Build history of the part. All positions in model axes, mm. A direction names the side the tool comes from. Round coordinates to 2 decimals unless told otherwise and drop trailing zeros. Write each loop counter-clockwise with the first axis right and the second up, starting at its lowest first coordinate (ties: lowest second). Pieces come first, ordered by that corner, then holes. Notation, with made-up numbers: (80.25, 67.25) -> (89.25, 67.25) arc R19 ccw to (89.25, 86.25) -> close; hole circle Ø4 at (2.25, 41.5). An arc over 180 degrees is marked (long way). Answer as CSV lines item,"result".
from build123d import *

# Parameters (mm, degrees)
SKETCH1_W           = 72.5
SKETCH1_H           = 72.5
SKETCH1_R           = 17.5
SKETCH1_R_2         = 2.125
BOSS_EXTRUDE1_DEPTH = 5
BOSS_EXTRUDE2_DEPTH = 50
SKETCH18_R          = 5
CUT_EXTRUDE1_DEPTH  = 2.5
BOSS_EXTRUDE3_DEPTH = 5.5
SKETCH8_W           = 72.5
SKETCH8_H           = 5
BOSS_EXTRUDE4_DEPTH = 54.5
BOSS_EXTRUDE5_DEPTH = 35
BOSS_EXTRUDE7_DEPTH = 1.25
SKETCH12_W          = 85.832523084
SKETCH12_H          = 136.148140064
SKETCH12_R          = 2.25
BOSS_EXTRUDE6_DEPTH = 5
FILLET10_R          = 0.5
SKETCH26_W          = 72.5
SKETCH26_H          = 36.25
CUT_EXTRUDE3_DEPTH  = 166.204098106


with BuildPart() as part:
    # Sketch1 → Boss-Extrude1 (new body)
    with BuildSketch(Plane.XY):
        with Locations((36.25, 36.25)):
            Rectangle(SKETCH1_W, SKETCH1_H)
        with Locations((36.25, 36.25)):
            Circle(SKETCH1_R, mode=Mode.SUBTRACT)
        with Locations((11.25, 61.25)):
            Circle(SKETCH1_R_2, mode=Mode.SUBTRACT)
        with Locations((61.25, 61.25)):
            Circle(SKETCH1_R_2, mode=Mode.SUBTRACT)
        with Locations((61.25, 11.25)):
            Circle(SKETCH1_R_2, mode=Mode.SUBTRACT)
        with Locations((11.25, 11.25)):
            Circle(SKETCH1_R_2, mode=Mode.SUBTRACT)
    extrude(amount=BOSS_EXTRUDE1_DEPTH)

    # Sketch18 → Cut-Extrude1 (cut)
    with BuildSketch(Plane.XY):
        with Locations((61.25, 61.25)):
            Circle(SKETCH18_R)
        with Locations((11.25, 61.25)):
            Circle(SKETCH18_R)
        with Locations((61.25, 11.25)):
            Circle(SKETCH18_R)
        with Locations((11.25, 11.25)):
            Circle(SKETCH18_R)
    extrude(amount=CUT_EXTRUDE1_DEPTH, mode=Mode.SUBTRACT)

    # Sketch7 → Boss-Extrude3 (add)
    with BuildSketch(Plane.XY.offset(5)):
        Polygon((0, 0), (72.5, 0), (72.5, 36.25), (66.35, 36.25), (66.35, 5), (6.15, 5), (6.15, 36.25), (0, 36.25), align=None)
    extrude(amount=BOSS_EXTRUDE3_DEPTH)



with BuildPart() as body_2:
    # Sketch5 → Boss-Extrude2 (new body)
    with BuildSketch(Plane.XY.offset(65)):
        with BuildLine():
            Line((0, 0), (72.5, 0))
            Line((72.5, 0), (72.5, 5))
            Line((72.5, 5), (61.25, 5))
            Line((61.25, 5), (61.25, 36.25))
            Line((61.25, 36.25), (58.5, 36.25))
            ThreePointArc((58.5, 36.25), (36.25, 14), (14, 36.25))
            Line((14, 36.25), (11.25, 36.25))
            Line((11.25, 36.25), (11.25, 5))
            Line((11.25, 5), (0, 5))
            Line((0, 5), (0, 0))
        make_face()
    extrude(amount=BOSS_EXTRUDE2_DEPTH)


with BuildPart() as part_1:
    add(part.part)

    add(body_2.part)  # Boss-Extrude4 merges body 2
    # Sketch8 → Boss-Extrude4 (add)
    with BuildSketch(Plane.XY.offset(65)):
        with Locations((36.25, 2.5)):
            Rectangle(SKETCH8_W, SKETCH8_H)
    extrude(amount=-BOSS_EXTRUDE4_DEPTH)

    # Sketch11 → Boss-Extrude5 (add)
    with BuildSketch(Plane.XY.offset(10.5)):
        with BuildLine():
            Line((0, 5), (29.147359646, 5))
            Line((29.147359646, 5), (29.147359646, 7))
            ThreePointArc((29.147359646, 7), (12.587799398, 17.645961119), (6.15, 36.25))
            Line((6.15, 36.25), (0, 36.25))
            Line((0, 36.25), (0, 5))
        make_face()
        with BuildLine():
            Line((72.5, 5), (43.352640354, 5))
            Line((43.352640354, 5), (43.352640354, 7))
            ThreePointArc((43.352640354, 7), (59.912200602, 17.645961119), (66.35, 36.25))
            Line((66.35, 36.25), (72.5, 36.25))
            Line((72.5, 36.25), (72.5, 5))
        make_face()
    extrude(amount=BOSS_EXTRUDE5_DEPTH)

    # Sketch17 → Boss-Extrude7 (add)
    with BuildSketch(Plane(origin=(0, 5, 0), x_dir=(1, 0, 0), z_dir=(0, 1, 0))):
        Polygon((6.15, -5), (6.15, -10.5), (66.465854546, -10.5), (66.35, -5), align=None)
    extrude(amount=BOSS_EXTRUDE7_DEPTH)

    # Sketch12 → Boss-Extrude6 (add)
    with BuildSketch(Plane(origin=(0, 0, 0), x_dir=(1, 0, 0), z_dir=(0, 1, 0))):
        with Locations((36.25, -57.5)):
            Rectangle(SKETCH12_W, SKETCH12_H)
        with Locations(Location((-2.666504617, 4.229628013, 0), (0, 0, 90))):
            Circle(SKETCH12_R, mode=Mode.SUBTRACT)
        with Locations(Location((75.166504617, 4.229628013, 0), (0, 0, 90))):
            Circle(SKETCH12_R, mode=Mode.SUBTRACT)
        with Locations(Location((75.166504617, -119.229628013, 0), (0, 0, 90))):
            Circle(SKETCH12_R, mode=Mode.SUBTRACT)
        with Locations(Location((-2.666504617, -119.229628013, 0), (0, 0, 90))):
            Circle(SKETCH12_R, mode=Mode.SUBTRACT)
    extrude(amount=BOSS_EXTRUDE6_DEPTH)

    # Fillet10
    fillet10_edges = [part_1.edges().sort_by_distance(p)[0] for p in [
        (29.147359646, 7, 28),
        (43.352640354, 7, 28),
    ]]
    fillet(fillet10_edges, radius=FILLET10_R)

    # Sketch26 → Cut-Extrude3 (cut, through all)
    with BuildSketch(Plane.XY):
        with Locations((36.25, 54.375)):
            Rectangle(SKETCH26_W, SKETCH26_H)
    extrude(amount=CUT_EXTRUDE3_DEPTH, mode=Mode.SUBTRACT)


solid = part_1.part
1. Which spindle directions (+Z, -Z, +X, -X, +Y, -Y) get a long thin tool onto all of the face, cutting with end or side? Do faces 1 (the cylindrical face through (9.56, 9.96, 3.73)), 2 (the flat face through (8, 17, 45.5)), 3 (the flat face through (11.25, 21, 90)), 4 (the cylindrical face through (12.64, 17.58, 27.76)). Say none if no direction does.
Results found:
face 1,"-Z"
face 2,"+X, -X, +Y"
face 3,"+Z, -X, +Y"
face 4,"+Y"
2. Drop flat-ended pins along their axis: pin 1 Ø11 at (x, y) = (9.5, 13) entering from -Z; pin 2 Ø2 at (x, z) = (38.5, 31.5) entering from +Y; pin 3 Ø5.5 at (x, y) = (61.25, 11.25) entering from -Z; pin 4 Ø5 at (x, z) = (75.17, 119.23) entering from -Y. Give the stop position or say it passes through.
Results found:
pin 1,"stops at z = 0"
pin 2,"stops at y = 5"
pin 3,"stops at z = 2.5"
pin 4,"stops at y = 0"
3. Mould opens along Z. For faces 5 (the flat face through (36, 2, -10.574)), 6 (the flat face through (61.25, 20, 90)), 7 (the flat face through (36, 5, 57)), 8 (the flat face through (12, 12, 10.5)) say: +Z half, -Z half, draft (parallel to the pull), parting line (faces both ways), or undercut.
Results found:
face 5,"-Z half"
face 6,"draft"
face 7,"undercut"
face 8,"undercut"
4. Cut at C-C, the plane z = 14. Write the cut outline in (x, y).
Results found:
outline,"(-6.67, 0) -> (79.17, 0) -> (79.17, 5) -> (72.5, 5) -> (72.5, 36.25) -> (66.35, 36.25) arc R30.1 cw to (43.73, 7.09) arc R0.5 ccw to (43.35, 6.61) -> (43.35, 5) -> (29.15, 5) -> (29.15, 6.61) arc R0.5 ccw to (28.77, 7.09) arc R30.1 cw to (6.15, 36.25) -> (0, 36.25) -> (0, 5) -> (-6.67, 5) -> close"
5. Cut at D-D, the plane x = 36.25. Write the cut outline in (y, z), then the cut area to 3 significant figures.
Results found:
outline,"(0, -10.57) -> (5, -10.57) -> (5, 0) -> (18.75, 0) -> (18.75, 5) -> (6.25, 5) -> (6.25, 10.5) -> (5, 10.5) -> (5, 65) -> (14, 65) -> (14, 115) -> (5, 115) -> (5, 125.57) -> (0, 125.57) -> close"
area,"1,210 mm2"
6. Cut at B-B, the plane x = 3. Write the cut outline in (y, z), then the cut area to 3 significant figures.
Results found:
outline,"(0, -10.57) -> (5, -10.57) -> (5, 0) -> (36.25, 0) -> (36.25, 45.5) -> (5, 45.5) -> (5, 125.57) -> (0, 125.57) -> close"
area,"2,100 mm2"
7. Cut at A-A, the plane y = 23. Write the cut outline in (x, z).
Results found:
outline,"(0, 0) -> (24.82, 0) -> (24.82, 5) -> (6.15, 5) -> (6.15, 10.5) -> (9.22, 10.5) -> (9.22, 45.5) -> (0, 45.5) -> close; (11.25, 65) -> (18.38, 65) -> (18.38, 115) -> (11.25, 115) -> close; (47.68, 0) -> (72.5, 0) -> (72.5, 45.5) -> (63.28, 45.5) -> (63.28, 10.5) -> (66.35, 10.5) -> (66.35, 5) -> (47.68, 5) -> close; (54.12, 65) -> (61.25, 65) -> (61.25, 115) -> (54.12, 115) -> close"
8. Probe line 1 along Z through (x, y) = (18, 10.5); line 2 along Z through (x, y) = (27, 11); line 3 along Y through (x, z) = (11, 4). List the from-to ranges inside material, lowest first.
Results found:
line 1,"z = 0 to 5, 10.5 to 45.5, 65 to 115"
line 2,"z = 0 to 5, 65 to 115"
line 3,"y = 0 to 9.14, 13.36 to 36.25"
